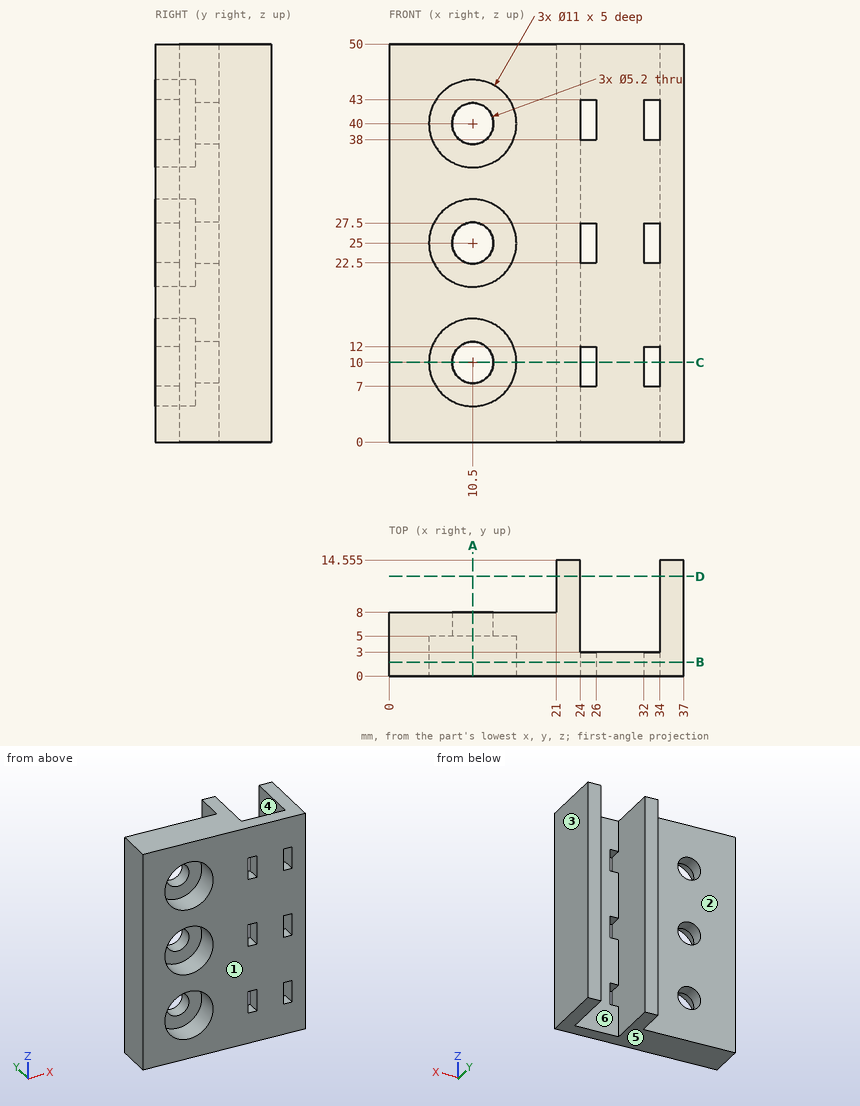
Study the drawing (mm; zero at the part's minimum x, y, z) and answer. A direction names the side the tool comes from. Give positions to 0.01 mm unless a question says otherwise; leave off trailing zeros. Order: outer loops, then holes, each group sorted by start corner. A loop starts at its lowest first (then second) coordinate and runs counter-clockwise, first axis right, second up.
1) Find section B-B on y = 1.75. Give the number of separate pieces and of enclosed holes in the cut face, then the cut area to 4 significant figures.
Reported:
separate pieces: 1
enclosed holes: 9
area: 1,505 mm2
2) Consider line 1 along Z through (x, y) = (10.5, 4); line 2 along X through (y, z) = (6.4, 10); line 3 along Z through (x, y) = (10.5, 6.45). Determine where each line is inside the solid, lowest interval first.
Reported:
line 1: z = 0 to 4.5, 15.5 to 19.5, 30.5 to 34.5, 45.5 to 50
line 2: x = 0 to 7.9, 13.1 to 24, 34 to 37
line 3: z = 0 to 7.4, 12.6 to 22.4, 27.6 to 37.4, 42.6 to 50
3) Find section D-D on y = 12.5. Write down the section's boundary in (x, z), then the cut area to 3 significant figures.
Reported:
outline: (21, 0) - (24, 0) - (24, 50) - (21, 50) - close; (34, 0) - (37, 0) - (37, 50) - (34, 50) - close
area: 300 mm2
4) Find section C-C on z = 10. Write down the section's boundary in (x, y) (1 decimal).
Reported:
outline: (0, 0) - (5, 0) - (5, 5) - (7.9, 5) - (7.9, 8) - (0, 8) - close; (13.1, 5) - (16, 5) - (16, 0) - (24, 0) - (24, 14.6) - (21, 14.6) - (21, 8) - (13.1, 8) - close; (26, 0) - (32, 0) - (32, 3) - (26, 3) - close; (34, 0) - (37, 0) - (37, 14.6) - (34, 14.6) - close
5) For the marked faces 1 and 2, determine the directions among +Z, -Z, +X, -X, +Y, -Y from which every point of the face is accessible in a straight line to the end or side of a thin tool.
Reported:
face 1: +Z, -Z, +X, -X, -Y
face 2: +Z, -Z, -X, +Y
6) Find section A-A on x = 10.5. Write down the section's boundary in (y, z), then the cut area to 3 significant figures.
Reported:
outline: (0, 0) - (8, 0) - (8, 7.4) - (5, 7.4) - (5, 4.5) - (0, 4.5) - close; (0, 15.5) - (5, 15.5) - (5, 12.6) - (8, 12.6) - (8, 22.4) - (5, 22.4) - (5, 19.5) - (0, 19.5) - close; (0, 30.5) - (5, 30.5) - (5, 27.6) - (8, 27.6) - (8, 37.4) - (5, 37.4) - (5, 34.5) - (0, 34.5) - close; (0, 45.5) - (5, 45.5) - (5, 42.6) - (8, 42.6) - (8, 50) - (0, 50) - close
area: 188 mm2
7) Given P1, Ø10, axis at x = 10.5, z = 25, coming from the -Y side; P2, Ø4.5, axis at x = 10.5, z = 10, coming from the +Y side; P3, Ø2, axis at y = 12, z = 17.5, coming from the -X side; P4, Ø6, axis at x = 10.5, z = 40, coming from the +Y side, each flat-ended and moving along its own axis, determine where each tip first touches the part or whether it passes through.
Reported:
P1: stops at y = 5
P2: passes through
P3: stops at x = 21
P4: stops at y = 8
8) Determine the mould class of the marked faces 3, 4, 5 and 6 for opening direction X: pulls with the +X half, pulls with the -X half, needs draft (parallel to the pull), parting line crosses it, or undercut.
Reported:
face 3: pulls with the +X half
face 4: undercut
face 5: needs draft
face 6: undercut
